```python
from build123d import *

# Parameters (mm, degrees)
SKETCH1_R               = 7.874
BOSS_EXTRUDE1_DEPTH     = 101.6
SKETCH2_R               = 6.35
BOSS_EXTRUDE2_DEPTH     = 38.1
CUT_EXTRUDE3_DEPTH      = 1.5875
CUT_EXTRUDE5_DEPTH      = 1.524
CUT_EXTRUDE5_DEPTH_BACK = 1.1684


with BuildPart() as part:
    # Sketch1 → Boss-Extrude1 (new body)
    with BuildSketch(Plane.XY):
        Circle(SKETCH1_R)
    extrude(amount=BOSS_EXTRUDE1_DEPTH)

    # Sketch2 → Boss-Extrude2 (add)
    with BuildSketch(Plane.XY.offset(101.6)):
        with Locations(Location((0, 0, 0), (0, 0, 180))):
            Circle(SKETCH2_R)
    extrude(amount=BOSS_EXTRUDE2_DEPTH)

    # Sketch6 → Cut-Extrude3 (cut)
    with BuildSketch(Plane(origin=(0, 6.35, 139.7), x_dir=(1, 0, 0), z_dir=(0, 1, 0))):
        with BuildLine():
            Line((1.5875, 33.02), (1.5875, 7.62))
            ThreePointArc((1.5875, 7.62), (0, 6.0325), (-1.5875, 7.62))
            Line((-1.5875, 7.62), (-1.5875, 33.02))
            ThreePointArc((-1.5875, 33.02), (0, 34.6075), (1.5875, 33.02))
        make_face()
    extrude(amount=-CUT_EXTRUDE3_DEPTH, mode=Mode.SUBTRACT)

    # Sketch7 → Cut-Extrude5 (cut, two sides: drawn at the far end of the back side and taken through both)
    with BuildSketch(Plane(origin=(0, 6.35, 139.7), x_dir=(1, 0, 0), z_dir=(0, 1, 0)).offset(-CUT_EXTRUDE5_DEPTH_BACK)):
        with BuildLine():
            Line((2.3876, 131.1275), (2.3876, 102.5525))
            ThreePointArc((2.3876, 102.5525), (0, 100.1649), (-2.3876, 102.5525))
            Line((-2.3876, 102.5525), (-2.3876, 131.1275))
            ThreePointArc((-2.3876, 131.1275), (0, 133.5151), (2.3876, 131.1275))
        make_face()
    extrude(amount=CUT_EXTRUDE5_DEPTH + CUT_EXTRUDE5_DEPTH_BACK, mode=Mode.SUBTRACT)


solid = part.part
```
For this review, take the finished solid that the model builds, in its own axes (mm). A direction names the side the tool comes from. Coordinates: 2 decimals unless noted, no trailing zeros. Write each loop counter-clockwise with the first axis right and the second up, starting at its lowest first coordinate (ties: lowest second). Pieces come first, ordered by that corner, then holes. Notation, with made-up numbers: (26.25, 67) -> (80.25, 67) arc R17 cw to (80.25, 96) -> close; hole circle Ø2 at (-0.5, -6). An arc over 180 degrees is marked (long way). Put each result on its own line as item: value.
Q1. Take a section at D-D, the plane z = 108.5. State the section outline as (x, y) points, then the cut area to 3 significant figures.
From the geometry:
outline: (-1.59, 4.76) -> (-1.59, 6.15) arc R6.35 ccw (long way) to (1.59, 6.15) -> (1.59, 4.76) -> close
area: 122 mm2
Q2. Take a section at A-A, the plane x = 0. State the section outline as (y, z) points, then the cut area to 3 significant figures.
From the geometry:
outline: (-7.87, 0) -> (7.87, 0) -> (7.87, 6.18) -> (5.18, 6.18) -> (5.18, 39.54) -> (7.87, 39.54) -> (7.87, 101.6) -> (6.35, 101.6) -> (6.35, 105.09) -> (4.76, 105.09) -> (4.76, 133.67) -> (6.35, 133.67) -> (6.35, 139.7) -> (-6.35, 139.7) -> (-6.35, 101.6) -> (-7.87, 101.6) -> close
area: 1,950 mm2
Q3. Tool access review of faces 1 (the flat face through (0, 5.182, 23)), 2 (the flat face through (0, 0, 139.7)): name each direction out of +Z, -Z, +X, -X, +Y, -Y from which nothing blocks a thin tool from reaching the whole face with its end or side.
From the geometry:
face 1: +Y
face 2: +Z, +X, -X, +Y, -Y
Q4. Clearance check with flat-ended pins moving along their axes: pin 1 Ø1 at (x, z) = (2, 23) entering from +Y; pin 2 Ø2.5 at (y, z) = (6.5, 28) entering from +X; pin 3 Ø2 at (y, z) = (-2, 19.5) entering from +X. State where each tip first meets the part, or that it passes through.
From the geometry:
pin 1: stops at y = 7.5
pin 2: stops at x = 5.87
pin 3: stops at x = 7.81
Q5. Take a section at C-C, the plane z = 19. State the section outline as (x, y) points, then the cut area to 3 significant figures.
From the geometry:
outline: (-2.39, 5.18) -> (-2.39, 7.5) arc R7.87 ccw (long way) to (2.39, 7.5) -> (2.39, 5.18) -> close
area: 183 mm2
Q6. Wall thickness on L1, parallel to Y at x = -0.5, z = 108.5; L2, parallel to Z at x = 5.5, y = 5.25; L3, parallel to X at y = -0.25, z = 56.5: over which ranges is each line inside the solid? List them lowest first.
From the geometry:
L1: y = -6.33 to 4.76
L2: z = 0 to 101.6
L3: x = -7.87 to 7.87
Q7. Take a section at B-B, the plane y = 0. State the section outline as (x, z) points, then the cut area to 3 significant figures.
From the geometry:
outline: (-7.87, 0) -> (7.87, 0) -> (7.87, 101.6) -> (6.35, 101.6) -> (6.35, 139.7) -> (-6.35, 139.7) -> (-6.35, 101.6) -> (-7.87, 101.6) -> close
area: 2,080 mm2
Q8. The part is to be moulded in two halves that separate along X. For faces 3 (the cylindrical face through (0.8, -6.3, 120.4)), 4 (the flat face through (0, 4.762, 119)), 5 (the flat face through (0.5, 6.5, 101.6)), say which applies: +X half, -X half, draft (parallel to the pull), parting line (faces both ways), or undercut.
From the geometry:
face 3: parting line
face 4: undercut
face 5: draft
